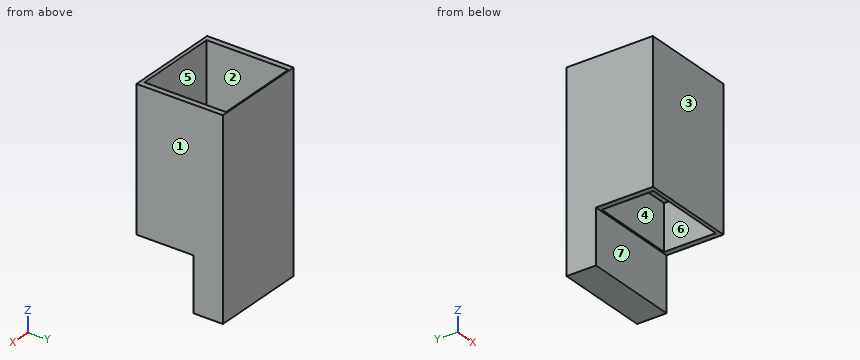
from build123d import *

# Parameters (mm, degrees)
BOSS_EXTRUDE1_DEPTH = 431.8
SKETCH2_W           = 381
SKETCH2_H           = 231.14
CUT_EXTRUDE1_DEPTH  = 203.2
SKETCH3_W           = 381
SKETCH3_H           = 365.76
CUT_EXTRUDE2_DEPTH  = 412.496


with BuildPart() as part:
    # Sketch1 → Boss-Extrude1 (new body)
    with BuildSketch(Plane(origin=(0, 0, 0), x_dir=(0, 0, -1), z_dir=(1, 0, 0))):
        Polygon((412.496, 387.35), (869.696, 387.35), (869.696, 255.27), (628.396, 255.27), (628.396, 0), (412.496, 0), (0, 0), (0, 387.35), align=None)
    extrude(amount=BOSS_EXTRUDE1_DEPTH)

    # Sketch2 → Cut-Extrude1 (cut)
    with BuildSketch(Plane(origin=(0, 0, -628.396), x_dir=(-1, 0, 0), z_dir=(0, 0, -1))):
        with Locations((-215.9, 132.08)):
            Rectangle(SKETCH2_W, SKETCH2_H)
    extrude(amount=-CUT_EXTRUDE1_DEPTH, mode=Mode.SUBTRACT)

    # Sketch3 → Cut-Extrude2 (cut)
    with BuildSketch(Plane.XY):
        with Locations((215.9, 199.39)):
            Rectangle(SKETCH3_W, SKETCH3_H)
    extrude(amount=-CUT_EXTRUDE2_DEPTH, mode=Mode.SUBTRACT)


solid = part.part
Design review of the part built by this model. Coordinates are the model's own, in mm. Face numbers are marked on the shaded views. A direction names the side the tool comes from. Coordinates: 2 decimals unless noted, no trailing zeros. Order: outer loops, then holes, each group sorted by start corner. A loop starts at its lowest first (then second) coordinate and runs counter-clockwise, first axis right, second up. Notation, with made-up numbers: M 18.5,23 L 35.5,23 A33 cw 35.5,52 Z; hole C -32,-35 d9. An arc over 180 degrees is marked long. Use a Markdown table: item, result.
(1) Draft analysis for pull direction X (two halves, no side actions). For the marked faces 1, 2, 3 and 4, state which applies: released by +X, released by -X, zero draft, split by the parting line, or undercut.
Worked answers:
| item | result |
|---|---|
| face 1 | released by +X |
| face 2 | undercut |
| face 3 | zero draft |
| face 4 | undercut |
(2) For P1, Ø10, axis at y = 253.5, z = -747.5, coming from the +X side; P2, Ø3, axis at x = 164.5, y = 63.5, coming from the -Z side; P3, Ø1, axis at x = 43.5, z = -722, coming from the -Y side, all flat-tipped, find the tip position at first contact; note any pin that passes through.
Worked answers:
| item | result |
|---|---|
| P1 | stops at x = 431.8 |
| P2 | stops at z = -425.2 |
| P3 | stops at y = 255.27 |
(3) For the marked faces 5, 6 and 7, list the 3-axis set-ups (+Z, -Z, +X, -X, +Y, -Y) from which the entire face can be reached by the end or side of a thin tool; tool diameter is ignored.
Worked answers:
| item | result |
|---|---|
| face 5 | +Z |
| face 6 | -Z |
| face 7 | -Z, +X, -X, -Y |
(4) Add section B-B (y = 313). Give the boundary of the cut face in (x, z).
Worked answers:
| item | result |
|---|---|
| outline | M 0,-869.7 L 431.8,-869.7 L 431.8,0 L 406.4,0 L 406.4,-412.5 L 25.4,-412.5 L 25.4,0 L 0,0 Z |
(5) Add section D-D (z = -57.5). Give the boundary of the cut face in (x, y), then the cut area to 3 significant figures.
Worked answers:
| item | result |
|---|---|
| outline | M 0,0 L 431.8,0 L 431.8,387.35 L 0,387.35 Z; hole M 25.4,16.51 L 406.4,16.51 L 406.4,382.27 L 25.4,382.27 Z |
| area | 27,900 mm2 |
(6) Add section A-A (z = -506). Give the boundary of the cut face in (x, y).
Worked answers:
| item | result |
|---|---|
| outline | M 0,0 L 431.8,0 L 431.8,387.35 L 0,387.35 Z; hole M 25.4,16.51 L 406.4,16.51 L 406.4,247.65 L 25.4,247.65 Z |
(7) Add section C-C (x = 214). Give the boundary of the cut face in (y, z).
Worked answers:
| item | result |
|---|---|
| outline | M 0,-628.4 L 16.51,-628.4 L 16.51,-425.2 L 247.65,-425.2 L 247.65,-628.4 L 255.27,-628.4 L 255.27,-869.7 L 387.35,-869.7 L 387.35,0 L 382.27,0 L 382.27,-412.5 L 16.51,-412.5 L 16.51,0 L 0,0 Z |
(8) Wall thickness on probe 1 along X at (y, z) = (19, -452); probe 2 along Y at (x, z) = (106, -522); probe 3 along Y at (x, z) = (95, -50): over which ranges is each line inside the solid? List them lowest first.
Worked answers:
| item | result |
|---|---|
| probe 1 | x = 0 to 25.4, 406.4 to 431.8 |
| probe 2 | y = 0 to 16.51, 247.65 to 387.35 |
| probe 3 | y = 0 to 16.51, 382.27 to 387.35 |
